Could you check a few things on this model? Use its own coordinates, in mm. Round coordinates to 2 decimals unless told otherwise and drop trailing zeros. Write each loop counter-clockwise with the first axis right and the second up, starting at its lowest first coordinate (ties: lowest second). Pieces come first, ordered by that corner, then holes. Notation, with made-up numbers: (-8.75, -9) -> (7.25, -9) arc R34 ccw to (7.25, 28) -> close; hole circle Ø7 at (-2.5, 32). An arc over 180 degrees is marked (long way). Answer as CSV lines item,"result". Start each with the question number.
Q1. If we mould it in two halves opening along X, with no side actions, what happens to faces 1 (the cylindrical face through (106.892, -3.944, 54.972)), 2 (the cylindrical face through (105.9, -4.06, 99.85)), 3 (the flat face through (48, -4, 48)), 4 (the flat face through (111, -3.94, 26.15))? For each: pulls with the +X half, pulls with the -X half, needs draft (parallel to the pull), parting line crosses it, or undercut.
Q2. If I drill on line 1 (X direction, y = -5, z = 61); line 2 (Z direction, x = 100, y = -3.75); line 3 (X direction, y = -6.5, z = 63), over which ranges is the centre line in solid material (lowest first)? Write a range as [from, to].
Q3. Will these pins go through, and if not, where does the flat tip stop? pin 1 Ø4 at (y, z) = (-3, 16.5) entering from +X; pin 2 Ø1.5 at (x, y) = (110.5, -3.5) entering from +Z; pin 3 Ø3 at (x, y) = (98.5, -4) entering from -Z.
Q4. Imagine slicing it at A-A on z = 77. Please give me the cut outline in (x, y).
Q5. Imagine slicing it at B-B on x = 22. Please give me the cut outline in (y, z).
Q6. Imagine slicing it at C-C on y = -1.5. Please give me the cut outline in (x, z), and give its area (3 significant figures).
Q7. Imagine slicing it at D-D on z = 57. Please give me the cut outline in (x, y).
from build123d import *

# Parameters (mm, degrees)
F0_R     = 12.5
F1_DEPTH = 8
F2_R     = 15
F3_R     = 15


with BuildPart() as f1:
    # F0 (on Front) → F1 (new body)
    with BuildSketch(Plane.XZ):
        Polygon((106.066017, 106.066017), (0, 0), (84.852814, 0), (148.492424, 63.63961), align=None)
        with Locations((109.601551, 67.175144)):
            Circle(F0_R, mode=Mode.SUBTRACT)
    extrude(amount=F1_DEPTH)

    # F2
    f2_edges = [f1.edges().sort_by_distance(p)[0] for p in [
        (106.066017, -4, 106.066017),
    ]]
    fillet(f2_edges, radius=F2_R)

    # F3
    f3_edges = [f1.edges().sort_by_distance(p)[0] for p in [
        (148.492424, -4, 63.63961),
    ]]
    fillet(f3_edges, radius=F3_R)


solid = f1.part
Checks:
1,face 1,"undercut"
1,face 2,"parting line crosses it"
1,face 3,"pulls with the -X half"
1,face 4,"pulls with the +X half"
2,line 1,"[61, 98.73], [120.47, 142.05]"
2,line 2,"[15.15, 59.17], [75.18, 98.57]"
2,line 3,"[63, 97.82], [121.38, 142.27]"
3,pin 1,"x = 103.35"
3,pin 2,"z = 99.39"
3,pin 3,"z = 12.15"
4,outline,"(77, -8) -> (101.87, -8) -> (101.87, 0) -> (77, 0) -> close; (117.33, -8) -> (135.13, -8) -> (135.13, 0) -> (117.33, 0) -> close"
5,outline,"(-8, 0) -> (0, 0) -> (0, 22) -> (-8, 22) -> close"
6,outline,"(0, 0) -> (84.85, 0) -> (137.89, 53.03) arc R15 ccw to (137.89, 74.25) -> (116.67, 95.46) arc R15 ccw to (95.46, 95.46) -> close; hole circle Ø25 at (109.6, 67.18)"
6,area,"6,610 mm^2"
7,outline,"(57, -8) -> (102.34, -8) -> (102.34, 0) -> (57, 0) -> close; (116.86, -8) -> (140.73, -8) -> (140.73, 0) -> (116.86, 0) -> close"
